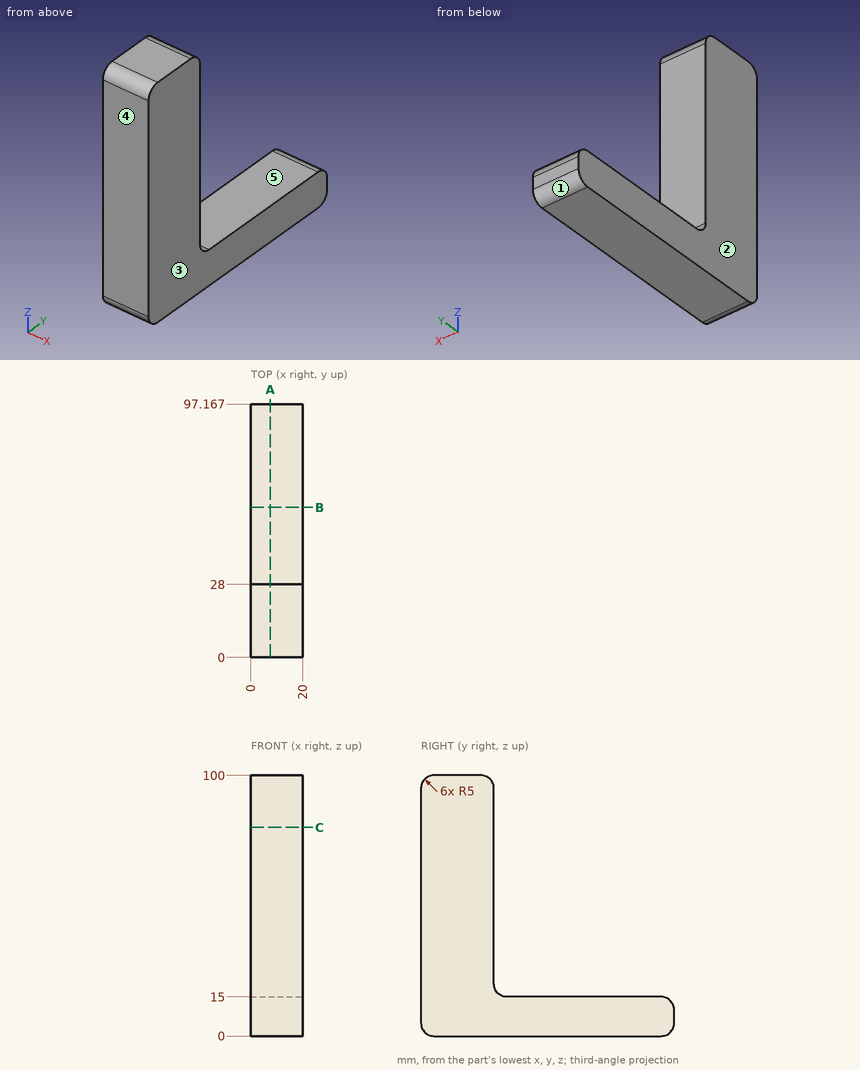
Source: three-view drawing plus pictorial views. Frame: mm from the lowest corner of the part. A direction names the side the tool comes from. Coordinates: 2 decimals unless noted, no trailing zeros. Order: outer loops, then holes, each group sorted by start corner. A loop starts at its lowest first (then second) coordinate and runs counter-clockwise, first axis right, second up. Notation, with made-up numbers: M 30.5,-1 L 63.5,-1 A35 ccw 63.5,33 Z; hole C 87,25.25 d4. An arc over 180 degrees is marked long. One line per question, with ' | ' between items.
Item 1: Draft query along X for the marked faces 1, 2 and 3. Return one class per face: released by +X, released by -X, zero draft, split by the parting line, or undercut.
Geometry results:
face 1: zero draft | face 2: released by -X | face 3: released by +X
Item 2: Section C-C (z = 80). Output: boundary loops of the cut face in (x, y).
Geometry results:
outline: M 0,0 L 20,0 L 20,28 L 0,28 Z
Item 3: Ray query, line 1 along Y through (x, z) = (19.25, 81); line 2 along Z through (x, y) = (2, 90.5); line 3 along Z through (x, y) = (17, 26). Return the intervals inside material, ascending.
Geometry results:
line 1: y = 0 to 28 | line 2: z = 0 to 15 | line 3: z = 0 to 99
Item 4: Reachability of the marked faces 4 and 5 from +Z, -Z, +X, -X, +Y, -Y: full face, straight path, thin tool, end or side. Return the list, or none.
Geometry results:
face 4: +Z, -Z, +X, -X, -Y | face 5: +Z, +X, -X, +Y
Item 5: Pin query (flat end, axial travel): pin 1 (1 mm diameter, centred on x = 16.5, z = 45.5, fed in from +Y); pin 2 (8 mm diameter, centred on x = 8, y = 77.5, fed in from +Z). Return the tip coordinate at first contact, or that it passes through.
Geometry results:
pin 1: stops at y = 28 | pin 2: stops at z = 15
Item 6: Section A-A (x = 7.5). Output: boundary loops of the cut face in (y, z).
Geometry results:
outline: M 0,5 A5 ccw 5,0 L 92.17,0 A5 ccw 97.17,5 L 97.17,10 A5 ccw 92.17,15 L 33,15 A5 cw 28,20 L 28,95 A5 ccw 23,100 L 5,100 A5 ccw 0,95 Z
Item 7: Section B-B (y = 57.5). Output: boundary loops of the cut face in (x, z).
Geometry results:
outline: M 0,0 L 20,0 L 20,15 L 0,15 Z
